```python
from build123d import *

# Parameters (mm, degrees)
F0_W     = 238.8670668006
F0_H     = 133.2817673683
F1_DEPTH = 80.772
F2_R     = 26.9812507731
F3_W     = 136.5834623575
F3_H     = 15.7284336165
F4_DEPTH = 15.748
F5_T     = 2.54


# Not quite as in the source:
# - a shell that OpenCascade refuses in one call is made with other operations: the cavity is built on its own and cut out


with BuildPart() as f1:
    # F0 (on Top) → F1 (new body)
    with BuildSketch(Plane.XY):
        with Locations((2.9073394835, 0.8117333055)):
            Rectangle(F0_W, F0_H)
    extrude(amount=F1_DEPTH)

    # F2
    f2_edges = [f1.edges().sort_by_distance(p)[0] for p in [
        (2.907339, -65.82915, 80.772),
        (2.907339, 67.452617, 80.772),
    ]]
    fillet(f2_edges, radius=F2_R)

    # F3 (on face) → F4 (join)
    with BuildSketch(Plane.XY.offset(80.772)):
        with Locations((-7.1703717113, 0.7790052332)):
            Rectangle(F3_W, F3_H)
    extrude(amount=F4_DEPTH)

    # F5: shell of thickness 2.54, made by hand


with BuildPart() as f5_core1:
    # F5_t2: copy of F1
    add(f1.part)

    # the walls: a layer under each face that stays
    f5_faces = [f5_core1.faces().sort_by_distance(p)[0] for p in [
        (2.9073394835, 67.4526169896, 26.8953746135),
        (122.3408728838, 0.8117333055, 40.386),
        (2.9073394835, 59.5499916031, 72.8693746135),
        (2.9073394835, 0.8117333055, 0),
        (-116.5261939168, 0.8117333055, 40.386),
        (2.9073394835, -65.8291503787, 26.8953746135),
        (2.9073394835, -57.9265249922, 72.8693746135),
        (-76.7150161167, -25.6280219686, 80.772),
    ]]
    thicken(f5_faces, amount=-F5_T, mode=Mode.SUBTRACT)


with BuildPart() as f1_1:
    add(f1.part)

    # what is left inside the walls is the cavity
    f5_cavity = [f5_core1.part.solids().sort_by_distance(p)[0] for p in [
        (2.907339, -20.555228, 2.5654),
    ]]
    add(f5_cavity, mode=Mode.SUBTRACT)


solid = f1_1.part
```
Read the model definition and answer for the solid it produces. Units are mm, in the model's axes. A direction names the side the tool comes from. Coordinates: 2 decimals unless noted, no trailing zeros. Loops run counter-clockwise (first coordinate to the right, second up) from the corner with the lowest first, then second, coordinate; pieces in that order, holes last.
(1) The part is cut by section A-A (x = 70.5). Determine the outline of the cut face in (y, z), and give its area (3 significant figures).
Solution:
outline: (-65.83, 0) - (67.45, 0) - (67.45, 53.79) arc R26.98 ccw to (40.47, 80.77) - (-38.85, 80.77) arc R26.98 ccw to (-65.83, 53.79) - close; hole (-63.29, 2.54) - (64.91, 2.54) - (64.91, 53.79) arc R24.44 ccw to (40.47, 78.23) - (-38.85, 78.23) arc R24.44 ccw to (-63.29, 53.79) - close
area: 1,010 mm2
(2) Flat-ended cylindrical pins translate along their axes: pin 1 Ø3 at (x, z) = (9.5, 79) entering from +Y; pin 2 Ø3 at (x, z) = (8, 79) entering from -Y; pin 3 Ø3 at (x, z) = (37, 60) entering from -Y (3 decimals). Find the tip coordinate at first contact, or state that the pin passes through.
Solution:
pin 1: stops at y = 53.35
pin 2: stops at y = -51.73
pin 3: stops at y = -65.415
(3) The part is cut by section B-B (z = 34.5). Determine the outline of the cut face in (x, y), and give its area (3 significant figures).
Solution:
outline: (-116.53, -65.83) - (122.34, -65.83) - (122.34, 67.45) - (-116.53, 67.45) - close; hole (-113.99, -63.29) - (119.8, -63.29) - (119.8, 64.91) - (-113.99, 64.91) - close
area: 1,860 mm2
(4) The mould has two halves that part along X. Classify faces 1 (the face through (1, -63.289, 28)), 2 (the face through (1, 67.453, 27)), 3 (the face through (-116.526, 0, 40)), 4 (the face through (122.341, 0, 40)): released by +X, released by -X, zero draft, split by the parting line, or undercut.
Solution:
face 1: undercut
face 2: zero draft
face 3: released by -X
face 4: released by +X
(5) The part is cut by section D-D (y = 6). Determine the outline of the cut face in (x, z).
Solution:
outline: (-116.53, 0) - (122.34, 0) - (122.34, 80.77) - (61.12, 80.77) - (61.12, 78.23) - (119.8, 78.23) - (119.8, 2.54) - (-113.99, 2.54) - (-113.99, 78.23) - (-75.46, 78.23) - (-75.46, 80.77) - (-116.53, 80.77) - close
(6) A tool of negligible diameter and unlimited length cuts with its end or side. For faces 5 (the face through (1, -65.829, 27)), 6 (the face through (1, 10, 78.232)), from which of +Z, -Z, +X, -X, +Y, -Y can it reach the whole face along a straight path? Write none if from no direction.
Solution:
face 5: +Z, -Z, +X, -X, -Y
face 6: none
(7) The part is cut by section C-C (y = -12). Determine the outline of the cut face in (x, z).
Solution:
outline: (-116.53, 0) - (122.34, 0) - (122.34, 80.77) - (-116.53, 80.77) - close; hole (-113.99, 2.54) - (119.8, 2.54) - (119.8, 78.23) - (-113.99, 78.23) - close
(8) Consider line 1 along Z through (x, y) = (87, -34); line 2 along X through (y, z) = (-5.5, 33); line 3 along Y through (x, z) = (26, 45.5). Determine where each line is inside the solid, lowest interval first.
Solution:
line 1: z = 0 to 2.54, 78.23 to 80.77
line 2: x = -116.53 to -113.99, 119.8 to 122.34
line 3: y = -65.83 to -63.29, 64.91 to 67.45
